Build history of the part. All positions in model axes, mm. A direction names the side the tool comes from. Give positions to 0.01 mm unless a question says otherwise; leave off trailing zeros. Loops run counter-clockwise (first coordinate to the right, second up) from the corner with the lowest first, then second, coordinate; pieces in that order, holes last. Notation, with made-up numbers: (-31.75, 18) -> (-14.75, 18) arc R23 cw to (-14.75, 51) -> close; hole circle Ø1 at (-22.75, 74.25). An arc over 180 degrees is marked (long way). One line per question, with ' | ' between items. Start each with the question number.
(1) Slice it at A-A, the plane x = 0. Write the cut outline in (y, z).
(2) 3-axis set-ups, long thin cutter, end or side, ignore diameter. For faces 1 (the face through (9.525, -3, -1)), 2 (the face through (-0.688, -9.481, -72.868)): which of +Z, -Z, +X, -X, +Y, -Y reach the whole face in a straight line?
(3) Flat gauge pins, fed straight in: pin 1 Ø3 at (x, y) = (-4, -10) entering from +Z; pin 2 Ø3 at (x, z) = (2.5, -29) entering from -Y; pin 3 Ø1 at (x, y) = (2, -7.5) entering from +Z; pin 4 Ø5 at (y, z) = (-11, 32) entering from -X. Where does each tip first touch, or does it go through?
(4) Drill centre line: L1, parallel to Y at x = 2.25, z = -43. Where is it in solid material? Low to high. Write a range as from..to.
(5) Mould opens along Z. For faces 3 (the face through (0, -6.35, 1)), 4 (the face through (-0.688, -9.481, 66.923)), 5 (the face through (-9.525, -3, -1)), 6 (the face through (0, -3, -76.2)) say: pulls with the +Z half, pulls with the -Z half, needs draft (parallel to the pull), parting line crosses it, or undercut.
(6) Slice it at B-B, the plane y = -8.75. Write the cut outline in (x, z) (3 decimals), then the cut area to 3 significant figures.
(7) Slice it at C-C, the plane z = 38.5. Write the cut outline in (x, y) (3 decimals).
```python
from build123d import *

# Parameters (mm, degrees)
F0_R     = 3.175
F0_W     = 19.05
F0_H     = 152.4
F1_DEPTH = 6.35
F2_DEPTH = 12.7


with BuildPart() as f1:
    # F0 (on Front) → F1 (new body)
    with BuildSketch(Plane.XZ):
        with Locations((0, 70.022136)):
            Circle(F0_R)
        Rectangle(F0_W, F0_H)
        with Locations((0, -69.768146)):
            Circle(F0_R, mode=Mode.SUBTRACT)
        with Locations((0, 70.022136)):
            Circle(F0_R, mode=Mode.SUBTRACT)
        with Locations((0, -69.768146)):
            Circle(F0_R)
    extrude(amount=F1_DEPTH)

    # F0 (on Front) → F2 (join)
    with BuildSketch(Plane.XZ):
        with Locations((0, 70.022136)):
            Circle(F0_R)
        with Locations((0, -69.768146)):
            Circle(F0_R)
    extrude(amount=F2_DEPTH)


solid = f1.part
```
Final values:
1) outline: (-12.7, -72.94) -> (-6.35, -72.94) -> (-6.35, -76.2) -> (0, -76.2) -> (0, 76.2) -> (-6.35, 76.2) -> (-6.35, 73.2) -> (-12.7, 73.2) -> (-12.7, 66.85) -> (-6.35, 66.85) -> (-6.35, -66.59) -> (-12.7, -66.59) -> close
2) face 1: +Z, -Z, +X, +Y, -Y | face 2: -Y
3) pin 1: z = 71.98 | pin 2: y = -6.35 | pin 3: z = 72.82 | pin 4: through
4) L1: -6.35..0
5) face 3: undercut | face 4: undercut | face 5: needs draft | face 6: pulls with the -Z half
6) outline: circle Ø6.35 at (0, -69.768); circle Ø6.35 at (0, 70.022) | area: 63.3 mm2
7) outline: (-9.525, -6.35) -> (9.525, -6.35) -> (9.525, 0) -> (-9.525, 0) -> close
